The drawing under review shows one solid part. Ordinate dimensions are in mm from its lowest x, y, z. A direction names the side the tool comes from. Give positions to 0.01 mm unless a question says otherwise; leave off trailing zeros. Order: outer loops, then holes, each group sorted by start corner. A loop starts at its lowest first (then second) coordinate and runs counter-clockwise, first axis right, second up. Notation, with made-up numbers: (-12, 14) - (25, 14) arc R31 ccw to (25, 41) - close; hole circle Ø7 at (87, 86.5). An arc over 180 degrees is marked (long way). Use CSV: the item, a comma, the result in double quotes.
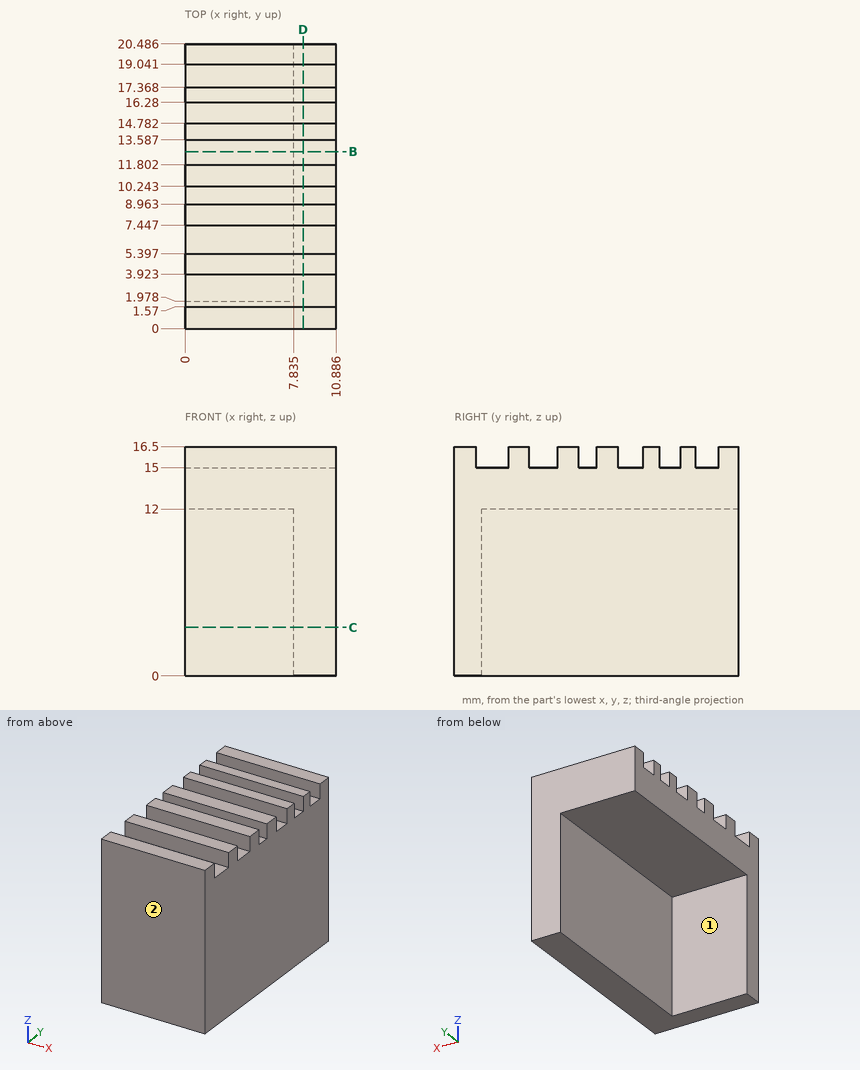
Item 1: Wall thickness on L1, parallel to Z at x = 1, y = 9.5; L2, parallel to Y at x = 7.25, z = 3.5; L3, parallel to X at y = 15.25, z = 10.5 (1 decimal): over which ranges is each line inside the solid? List them lowest first.
Results list:
L1,"z = 12 to 15"
L2,"y = 0 to 1.98"
L3,"x = 7.8 to 10.9"
Item 2: Clearance check with flat-ended pins moving along their axes: pin 1 (6 mm diameter, centred on x = 1.5, y = 10, fed in from -Z); pin 2 (1 mm diameter, centred on x = 5, z = 5.5, fed in from +Y). State where each tip first meets the part, or that it passes through.
Results list:
pin 1,"stops at z = 12"
pin 2,"stops at y = 1.98"
Item 3: Tool access review of the marked faces 1 and 2: name each direction out of +Z, -Z, +X, -X, +Y, -Y from which nothing blocks a thin tool from reaching the whole face with its end or side.
Results list:
face 1,"-Z, -X, +Y"
face 2,"+Z, -Z, +X, -X, -Y"
Item 4: Take a section at C-C, the plane z = 3.5. Give the boundary of the cut face in (x, y) (1 decimal).
Results list:
outline,"(0, 0) - (10.9, 0) - (10.9, 20.5) - (7.8, 20.5) - (7.8, 2) - (0, 2) - close"
Item 5: Take a section at B-B, the plane y = 12.75. Give the boundary of the cut face in (x, z) (1 decimal).
Results list:
outline,"(0, 12) - (7.8, 12) - (7.8, 0) - (10.9, 0) - (10.9, 15) - (0, 15) - close"
Item 6: Take a section at D-D, the plane x = 8.5. Give the boundary of the cut face in (y, z) (1 decimal).
Results list:
outline,"(0, 0) - (20.5, 0) - (20.5, 16.5) - (19, 16.5) - (19, 15) - (17.4, 15) - (17.4, 16.5) - (16.3, 16.5) - (16.3, 15) - (14.8, 15) - (14.8, 16.5) - (13.6, 16.5) - (13.6, 15) - (11.8, 15) - (11.8, 16.5) - (10.2, 16.5) - (10.2, 15) - (9, 15) - (9, 16.5) - (7.4, 16.5) - (7.4, 15) - (5.4, 15) - (5.4, 16.5) - (3.9, 16.5) - (3.9, 15) - (1.6, 15) - (1.6, 16.5) - (0, 16.5) - close"
